Can you work these out from the model? Positions are in its coordinate system, mm. Face numbers are marked on the shaded views. A direction names the side the tool comes from. Give positions to 0.01 mm unless a question says otherwise; leave off trailing zeros. Order: outer loops, then holes, each group sorted by start corner. A loop starts at its lowest first (then second) coordinate and runs counter-clockwise, first axis right, second up.
Item 1: If we mould it in two halves opening along X, with no side actions, what happens to the marked faces 1, 2 and 3? For each: +X half, -X half, draft (parallel to the pull), parting line (faces both ways), or undercut.
Item 2: If I drill on line 1 along Y through (x, z) = (-87.5, 0.35); line 2 along X through (y, z) = (24.5, -3.05); line 3 along X through (y, z) = (24.5, 0.1), over which ranges is the centre line in solid material (lowest first)?
Item 3: I want a section at A-A, the plane x = -20.5. Write out the boundary of the cut face in (y, z), then the cut area to 3 significant figures.
Item 4: I want a section at B-B, the plane x = -107.5. Write out the boundary of the cut face in (y, z).
Item 5: I'm going to push flat-ended pins straight in: pin 1 Ø3 at (y, z) = (2, 13.5) entering from +X; pin 2 Ø5 at (x, y) = (-1.5, 11) entering from -Z; pin 3 Ø16 at (y, z) = (-18, 13.5) entering from -X; pin 4 Ø19 at (x, y) = (0, -11.5) entering from +Z. Where does each tip first touch, or does it pass through?
Item 6: Which directions (+Z, -Z, +X, -X, +Y, -Y) give clear straight access to the entire face, cutting with the end or side of a thin tool? Please do the marked faces 4, 5 and 6.
Item 7: I want a section at C-C, the plane z = 24. Write out the boundary of the cut face in (x, y), then the cut area to 3 significant figures.
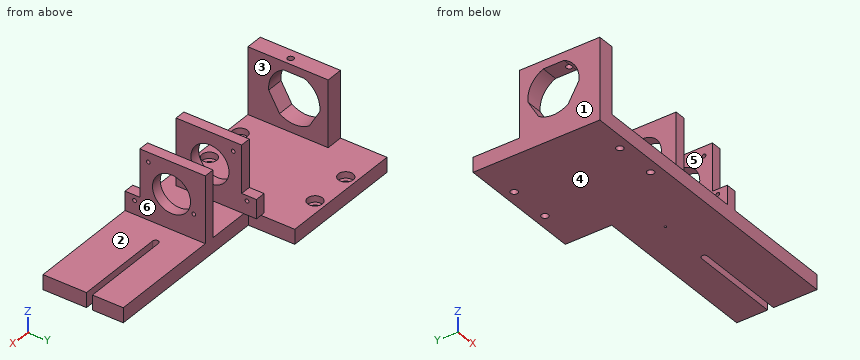
Autodesk Inventor part; units mm, degrees
ref_plane "Work Plane12" through (-127.4584, -23.859, -5) normal (0, 0, 1) x (1, 0, 0)
ref_plane "Work Plane14" through (-127.4584, -23.859, -5) normal (0, 0, 1) x (1, 0, 0)
ref_plane "YZ Plane" through (0, 0, 0) normal (1, 0, 0) x (0, 1, 0)
ref_plane "Work Plane10" through (-44.5, -14.2241, 18.7548) normal (1, 0, 0) x (0, -0.9087, 0.4175)
ref_plane "Work Plane11" through (-44.5, -8.5, 18.5) normal (-1, 0, 0) x (0, -1, 0)
sketch "Sketch9" plane through (-44.5, -8.5, 18.5) normal (-1, 0, 0) x (0, -1, 0)
  line L0 (16.8555, -12.7) -> (20, -12.7) construction
  circle A0 centre (17.5, -10) radius 1 construction
  circle A1 centre (11, 10.5) radius 1 construction
  circle A2 centre (-10.5, -5) radius 1 construction
  circle A3 centre (0, 0) radius 2.4142 construction
  line L1 (-15, 15) -> (15, 15) construction
  line L2 (16, -16) -> (-16, -16) construction
  line L3 (15, 15) -> (15, -15) construction
  line L4 (16, 16) -> (16, -16) construction
  line L5 (-16, -16) -> (-16, 16) construction
  line L6 (15, 15) -> (-16, 15)
  line L7 (-16, 15) -> (-16, -16.5)
  line L8 (-16, -16.5) -> (15, -16.5)
  line L9 (15, -16.5) -> (15, 15)
  circle A4 centre (11, 10.5) radius 0.9
  circle A5 centre (17.5, -10) radius 0.9
  circle A6 centre (-10.5, -5) radius 0.9
  circle A7 centre (0, 0) radius 9
  line L10 (15, -16.5) -> (22, -16.5)
  line L11 (22, -16.5) -> (22, -7.5)
  line L12 (22, -7.5) -> (15, -7.5)
  line L13 (15, -7.5) -> (15, -16.5)
  point P0 (-8.5, -18.5)
  dimension "d34" = 31.5
  dimension "d35" = 1.8
  dimension "d36" = 1.8
  dimension "d37" = 1.8
  dimension "d38" = 18
  dimension "d39" = 7
  dimension "d40" = 9
extrude "Extrusion7" add sketch "Sketch9" against normal blind 5
ref_plane "Work Plane12" through (-127.4584, -23.859, -5) normal (0, 0, 1) x (1, 0, 0)
sketch "Sketch10" plane through (-44.5, -30.5, 2) normal (0, 0, -1) x (-1, 0, 0)
  line L0 (0, 0) -> (0, 38)
  line L1 (0, 38) -> (-5, 38)
  line L2 (-5, 0) -> (-5, 38)
  line L3 (0, 0) -> (-5, 0)
  circle A0 centre (-19, 22) radius 1.4
  circle A1 centre (-57, 22) radius 1.4
  line L4 (82.9584, 8.641) -> (82.9584, 51.641)
  line L5 (-58.4, 38) -> (82.9584, 38)
  line L6 (82.9584, 38) -> (82.9584, 0)
  line L7 (82.9584, 0) -> (-58.4, 0)
  line L8 (-58.4, 0) -> (-58.4, 38)
  line L9 (-63.3254, 22) -> (-14.2903, 22) construction
  line L10 (-61.7754, 20.45) -> (-15.8403, 20.45)
  line L11 (-15.8403, 23.55) -> (-61.7754, 23.55)
  arc A2 (-61.7754, 23.55) -> (-61.7754, 20.45) centre (-61.7754, 22) ccw
  arc A3 (-15.8403, 20.45) -> (-15.8403, 23.55) centre (-15.8403, 22) ccw
  point P0 (-44.5, 30.5)
  point P1 (-38.8079, 22)
  dimension "d43" = 3.1
extrude "Extrusion8" add sketch "Sketch10" along normal up to surface (7 mm away) contours L3 L2 L1 L0 | L0 L5 L4 L6 L7 | L7 L8 L10 A3 L11 L5 L2 | L8 L11 A3 L10
sketch "Sketch11" plane through (-44.5, -30.5, -5) normal (0, 0, -1) x (-1, 0, 0)
  circle A0 centre (-57, 22) radius 1.4
  circle A1 centre (-19, 22) radius 1.4
  line L0 (-61.4468, 22) -> (-14.0111, 22) construction
  line L1 (-60.0468, 20.6) -> (-15.4111, 20.6)
  line L2 (-15.4111, 23.4) -> (-60.0468, 23.4)
  arc A2 (-60.0468, 23.4) -> (-60.0468, 20.6) centre (-60.0468, 22) ccw
  arc A3 (-15.4111, 20.6) -> (-15.4111, 23.4) centre (-15.4111, 22) ccw
  point P0 (-44.5, 30.5)
  point P1 (-58.4, 22)
  point P2 (-37.729, 22)
extrude "Extrusion9" cut sketch "Sketch11" against normal through all contours A0 | A0 L2 A1 L1 | A0 L1 A2 L2 | L2 A3 L1 A1
ref_plane "Work Plane13" through (-99.5, -8.5, 18.5) normal (-1, 0, 0) x (0, 0, 1)
sketch "Sketch12" plane through (-127.4584, -8.5, 18.5) normal (-1, 0, 0) x (0, 0, 1)
  circle A0 centre (0, 0) radius 10.125
  line L0 (-31.5, -12.684) -> (-23.5, -12.684)
  line L1 (-1.4, 6.6) -> (-6.6, 6.6)
  line L2 (-23.5, -22) -> (-23.5, 16)
  line L3 (-16.5, -22) -> (-23.5, -22)
  line L4 (-16.5, 16) -> (-16.5, -22)
  line L5 (-16.5, 16) -> (-23.5, 16)
  line L6 (15, 15) -> (15, -15)
  line L7 (-16.5, -22) -> (15, -22)
  line L8 (15, -22) -> (15, 16)
  line L9 (15, 16) -> (-16.5, 16)
  line L10 (-16.5, 16) -> (-16.5, -22)
  circle A1 centre (0, 0) radius 11.1
  line L11 (11.1, -5.0801) -> (11.1, 4.7426)
  line L12 (-1.1505, -12.1529) -> (-10.0048, -7.0409)
  line L13 (-10.0048, 7.0409) -> (-1.4428, 11.9842)
  arc A2 (-1.1505, -12.1529) -> (11.1, -5.0801) centre (0, 0) ccw
  arc A3 (11.1, 4.7426) -> (-1.4428, 11.9842) centre (0, 0) ccw
  arc A4 (-10.0048, 7.0409) -> (-10.0048, -7.0409) centre (0, 0) ccw
  point P0 (-18.5, 8.5)
  dimension "d51" = 60
  dimension "d52" = 60
  dimension "d73" = 22.2
extrude "Extrusion10" add sketch "Sketch12" against normal blind 8 contours L4 L9 L8 L6 L7
sketch "Sketch13" plane through (-127.4584, -30.5, 33.5) normal (0, 0, 1) x (-1, 0, 0)
  line L0 (0, -38) -> (0, 0)
  line L1 (0, -38) -> (-8, -38)
  line L2 (-8, -38) -> (-8, 0)
  line L3 (0, 0) -> (-8, 0)
  line L4 (6.7208, 32.125) -> (-12.4892, 32.125)
  circle A0 centre (-4.6991, -17.8249) radius 1.45
  point P0 (-127.4584, -30.5)
  dimension "d55" = 2.9
extrude "Extrusion11" cut sketch "Sketch13" against normal blind 8 contours A0
sketch "Sketch14" plane through (-44.5, -30.5, 2) normal (0, 0, 1) x (1, 0, 0)
  circle A0 centre (-63, 55) radius 1.45
  circle A1 centre (-43, 55) radius 1.45
  line L0 (-82.9584, 38) -> (-74.9584, 38)
  line L1 (-82.9584, 38) -> (58.4, 38)
  line L2 (-82.9584, 38) -> (-22.9584, 38)
  line L3 (-22.9584, 38) -> (-22.9584, 60)
  line L4 (-22.9584, 60) -> (-82.9584, 60)
  line L5 (-82.9584, 60) -> (-82.9584, 38)
  point P0 (44.5, 30.5)
  dimension "d71" = 60
  dimension "d72" = 22
ref_plane "Work Plane14" through (-127.4584, -23.859, -5) normal (0, 0, 1) x (1, 0, 0)
extrude "Extrusion12" add sketch "Sketch14" against normal up to surface (7 mm away)
sketch "Sketch15" plane through (-44.5, -30.5, 2) normal (0, 0, 1) x (1, 0, 0)
  line L0 (0, 38) -> (-22.9584, 38)
  line L1 (-82.9584, 60) -> (-82.9584, 38)
  line L2 (-74.9584, 0) -> (0, 0)
  line L3 (0, 0) -> (0, 38)
  line L4 (58.4, 20.6) -> (15.4111, 20.6)
  arc A0 (15.4111, 23.4) -> (15.4111, 20.6) centre (15.4111, 22) ccw
  line L5 (15.4111, 23.4) -> (58.4, 23.4)
  line L6 (58.4, 23.4) -> (58.4, 38)
  line L7 (5, 0) -> (5, 38)
  line L8 (5, 0) -> (58.4, 0)
  line L9 (58.4, 0) -> (58.4, 20.6)
  line L10 (-22.9584, 38) -> (-22.9584, 60)
  line L11 (-22.9584, 60) -> (-82.9584, 60)
  circle A1 centre (-63, 5) radius 1.45
  circle A2 centre (-43, 5) radius 1.45
  circle A3 centre (-43, 55) radius 1.45
  circle A4 centre (-63, 55) radius 1.45
  line L12 (58.4, 38) -> (5, 38)
  line L13 (-74.9584, 38) -> (-74.9584, 0)
  line L14 (-74.9584, 38) -> (-82.9584, 38)
  point P0 (44.5, 30.5)
  point P1 (-42.9584, 11.641)
  point P2 (-62.9584, 11.641)
hole "Hole3" at (-107.5, -25.5, 2) at (-87.5, -25.5, 2) at (-107.5, 24.5, 2) at (-87.5, 24.5, 2) direction (0, 0, -1) diameter 3.3 end through all counterbore diameter 7 counterbore depth 3
ref_plane "Work Plane15" through (-53.5, -8.5, 18.5) normal (-1, 0, 0) x (0, 0, 1)
sketch "Sketch17" plane through (-44.5, -30.5, 2) normal (0, 0, 1) x (1, 0, 0)
  circle A0 centre (-63, 55) radius 3.5
  circle A1 centre (-63, 5) radius 3.5
  circle A2 centre (-43, 5) radius 3.5
  circle A3 centre (-43, 55) radius 3.5
  line L0 (-74.9584, 0) -> (0, 0)
  line L1 (0, 0) -> (0, 38)
  line L2 (0, 38) -> (-22.9584, 38)
  line L3 (-22.9584, 38) -> (-22.9584, 60)
  line L4 (-22.9584, 60) -> (-82.9584, 60)
  line L5 (-82.9584, 60) -> (-82.9584, 38)
  line L6 (5, 31) -> (5, 13)
  line L7 (0, 13) -> (0, 31)
  circle A4 centre (-10, 22) radius 0.5
  line L8 (58.4, 20.6) -> (15.4111, 20.6)
  arc A5 (15.4111, 23.4) -> (15.4111, 20.6) centre (15.4111, 22) ccw
  line L9 (15.4111, 23.4) -> (58.4, 23.4)
  line L10 (58.4, 23.4) -> (58.4, 38)
  line L11 (5, 0) -> (5, 38)
  line L12 (5, 0) -> (58.4, 0)
  line L13 (58.4, 0) -> (58.4, 20.6)
  line L14 (58.4, 38) -> (5, 38)
  line L15 (-74.9584, 38) -> (-74.9584, 0)
  line L16 (-74.9584, 38) -> (-82.9584, 38)
  point P0 (44.5, 30.5)
  dimension "d78" = 1
  dimension "d85" = 10
extrude "Extrusion14" cut sketch "Sketch17" against normal blind 10 contours A4
pattern_circular "Circular Pattern1" count 2 over 360 about axis through (-54.5, -8.5, 2) along (0, 0, -1) of "Extrusion7"
properties part number "cellSTORM_inverted_Laser_10x_laserscanner_left_v2"
Results list:
1. face 1: -X half
1. face 2: draft
1. face 3: undercut
2. line 1: y = -30.5 to -29, -22 to 21, 28 to 29.5
2. line 2: x = -127.46 to -109.15, -105.85 to -89.15, -85.85 to -67.46
2. line 3: x = -127.46 to -111, -104 to -91, -84 to -67.46
3. outline: (-30.5, -5) - (-9.9, -5) - (-9.9, 2) - (-30.5, 2) - close; (-7.1, -5) - (7.5, -5) - (7.5, 2) - (-7.1, 2) - close
3. area: 246 mm2
4. outline: (-30.5, -5) - (-27.15, -5) - (-27.15, -1) - (-29, -1) - (-29, 2) - (-30.5, 2) - close; (-23.85, -5) - (22.85, -5) - (22.85, -1) - (21, -1) - (21, 2) - (-22, 2) - (-22, -1) - (-23.85, -1) - close; (26.15, -5) - (29.5, -5) - (29.5, 2) - (28, 2) - (28, -1) - (26.15, -1) - close
5. pin 1: stops at x = -39.5
5. pin 2: passes through
5. pin 3: stops at x = -127.46
5. pin 4: stops at z = 2
6. face 4: -Z, +X, -X, +Y, -Y
6. face 5: +Z, +Y, -Y
6. face 6: +Z, +X, +Y, -Y
7. outline: (-127.46, -30.5) - (-119.46, -30.5) - (-119.46, -19.4) - (-127.46, -19.4) - close; (-127.46, 2.24) - (-119.46, 2.24) - (-119.46, 7.5) - (-127.46, 7.5) - close; (-69.5, -24.5) - (-64.5, -24.5) - (-64.5, -15.62) - (-69.5, -15.62) - close; (-69.5, -1.38) - (-64.5, -1.38) - (-64.5, 6.5) - (-69.5, 6.5) - close; (-44.5, -23.5) - (-39.5, -23.5) - (-39.5, -15.62) - (-44.5, -15.62) - close; (-44.5, -1.38) - (-39.5, -1.38) - (-39.5, 7.5) - (-44.5, 7.5) - close
7. area: 298 mm2
